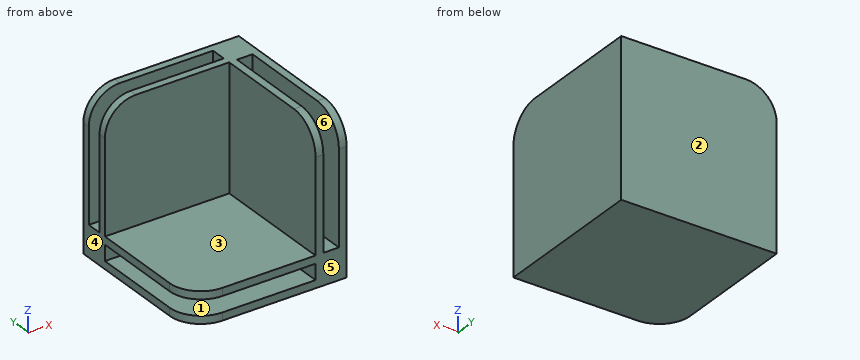
```python
from build123d import *

# Parameters (mm, degrees)
F1_DEPTH = 10
F3_DEPTH = 10
F5_DEPTH = 10
F6_W     = 20
F6_H     = 5
F6_W_2   = 5
F6_H_2   = 30
F6_H_3   = 20
F7_DEPTH = 40
F8_W     = 30
F8_H     = 5
F8_W_2   = 20
F9_DEPTH = 40


# Not quite as in the source:
# - a feature names something its author has since deleted; it is built from what else it names


with BuildPart() as f1:
    # F0 (on Top) → F1 (new body)
    with BuildSketch(Plane.XY):
        with BuildLine():
            Line((0, -50), (0, 0))
            Line((0, 0), (-50, 0))
            Line((-50, 0), (-50, -40))
            ThreePointArc((-50, -40), (-47.0710678119, -47.0710678119), (-40, -50))
            Line((-40, -50), (0, -50))
        make_face()
    extrude(amount=F1_DEPTH)

    # F2 (on Right) → F3 (join)
    with BuildSketch(Plane.YZ):
        with BuildLine():
            Line((-50, 10), (0, 10))
            Line((0, 10), (0, 50))
            Line((0, 50), (-40, 50))
            ThreePointArc((-40, 50), (-47.0710678119, 47.0710678119), (-50, 40))
            Line((-50, 40), (-50, 10))
        make_face()
    extrude(amount=-F3_DEPTH)

    # F4 (on Front) → F5 (join)
    with BuildSketch(Plane.XZ):
        with BuildLine():
            Line((-50, 10), (-10, 10))
            Line((-10, 10), (-10, 50))
            Line((-10, 50), (-40, 50))
            ThreePointArc((-40, 50), (-47.0710678119, 47.0710678119), (-50, 40))
            Line((-50, 40), (-50, 10))
        make_face()
    extrude(amount=F5_DEPTH)

    # F6 (on face) → F7 (cut)
    with BuildSketch(Plane.XZ.offset(50)):
        Polygon((-15, 2.5), (-10, 2.5), (-10, 7.5), (-40, 7.5), (-40, 2.5), align=None)
        with Locations((-50, 5)):
            Rectangle(F6_W, F6_H)
        with Locations((-5, 25)):
            Rectangle(F6_W_2, F6_H_2)
        with Locations((-5, 50)):
            Rectangle(F6_W_2, F6_H_3)
    extrude(amount=-F7_DEPTH, mode=Mode.SUBTRACT)

    # F8 (on face) → F9 (cut)
    with BuildSketch(Plane.XY.offset(50)):
        with Locations((-25, -5)):
            Rectangle(F8_W, F8_H)
        with Locations((-50, -5)):
            Rectangle(F8_W_2, F8_H)
    extrude(amount=-F9_DEPTH, mode=Mode.SUBTRACT)


solid = f1.part
```
Design review of the part built by this model. Coordinates are the model's own, in mm. Face numbers are marked on the shaded views. A direction names the side the tool comes from. Coordinates: 2 decimals unless noted, no trailing zeros. Order: outer loops, then holes, each group sorted by start corner. A loop starts at its lowest first (then second) coordinate and runs counter-clockwise, first axis right, second up. Notation, with made-up numbers: (-26, 52) - (20, 52) arc R22 cw to (20, 60) - close; hole circle Ø8 at (44, 41.25). An arc over 180 degrees is marked (long way). One line per question, with ' | ' between items.
Q1. To check wall thickness, follow line 1 along Z through (x, y) = (-16, -44); line 2 along Y through (x, z) = (-36, 15). State the ranges of each line that lie inside material, in increasing order.
Answer key:
line 1: z = 0 to 2.5, 7.5 to 10 | line 2: y = -10 to -7.5, -2.5 to 0
Q2. For the marked faces 1, 2 and 3, list the 3-axis set-ups (+Z, -Z, +X, -X, +Y, -Y) from which the entire face can be reached by the end or side of a thin tool; tool diameter is ignored.
Answer key:
face 1: -X, -Y | face 2: +Z, -Z, +X, -X, +Y | face 3: +Z, -X, -Y
Q3. The part is to be moulded in two halves that separate along X. For the marked faces 4, 5 and 6, say which applies: +X half, -X half, draft (parallel to the pull), parting line (faces both ways), or undercut.
Answer key:
face 4: -X half | face 5: draft | face 6: undercut
Q4. Clearance check with flat-ended pins moving along their axes: pin 1 Ø1 at (x, z) = (-39, 14.5) entering from -Y; pin 2 Ø1.5 at (y, z) = (-34.5, 43) entering from -X; pin 3 Ø1.5 at (x, y) = (-4, -21) entering from +Z. State where each tip first meets the part, or that it passes through.
Answer key:
pin 1: stops at y = -10 | pin 2: stops at x = -10 | pin 3: stops at z = 10
Q5. Consider section B-B, the plane z = 6. Give the boundary of the cut face in (x, y), then the cut area to 3 significant figures.
Answer key:
outline: (-50, -10) - (-10, -10) - (-10, -50) - (0, -50) - (0, 0) - (-50, 0) - close | area: 900 mm2
Q6. Consider section D-D, the plane x = -5. Give the boundary of the cut face in (y, z).
Answer key:
outline: (-50, 0) - (0, 0) - (0, 50) - (-10, 50) - (-10, 10) - (-50, 10) - close
Q7. Consider section A-A, the plane x = -14. Give the boundary of the cut face in (y, z).
Answer key:
outline: (-50, 0) - (0, 0) - (0, 50) - (-2.5, 50) - (-2.5, 10) - (-7.5, 10) - (-7.5, 50) - (-10, 50) - (-10, 10) - (-50, 10) - (-50, 7.5) - (-10, 7.5) - (-10, 2.5) - (-50, 2.5) - close
